Could you check a few things on this model? Use its own coordinates, in mm. Face numbers are marked on the shaded views. A direction names the side the tool comes from. Give positions to 0.01 mm unless a question says otherwise; leave off trailing zeros. Loops run counter-clockwise (first coordinate to the right, second up) from the corner with the lowest first, then second, coordinate; pieces in that order, holes last. Notation, with made-up numbers: M 81.5,12.25 L 113.5,12.25 A32 ccw 113.5,43.25 Z; hole C 80.5,62.25 d4. An arc over 180 degrees is marked long. Use CSV: the item, a comma, the result in double quotes.
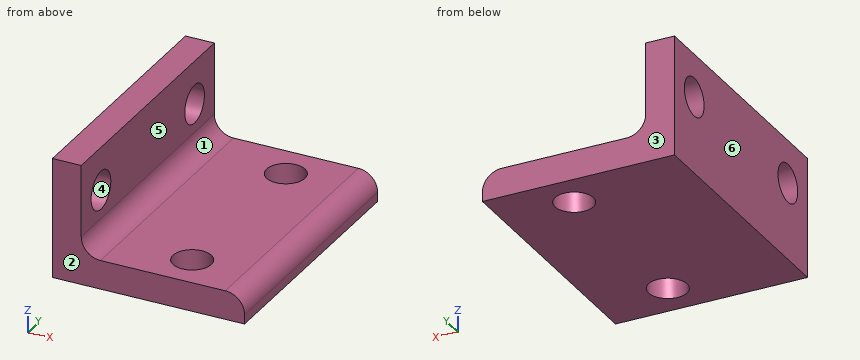
```python
from build123d import *

# Parameters (mm, degrees)
F1_DEPTH = 54
F2_R     = 4
F4_D     = 8
F4_DEPTH = 25
F6_D     = 8
F6_DEPTH = 25


with BuildPart() as f1:
    # F0 (on Front) → F1 (new body)
    with BuildSketch(Plane.XZ):
        Polygon((0, 25), (0, 0), (40, 0), (40, 6), (6, 6), (6, 25), align=None)
    extrude(amount=F1_DEPTH)

    # F2
    f2_edges = [f1.edges().sort_by_distance(p)[0] for p in [
        (40, -27, 6),
        (6, -27, 6),
    ]]
    fillet(f2_edges, radius=F2_R)

    # F4
    with Locations(Plane(origin=(0, 0, 0), x_dir=(0, -1, 0), z_dir=(-1, 0, 0))):
        with Locations((8, 16), (46, 16)):
            Hole(F4_D / 2, depth=F4_DEPTH)

    # F6
    with Locations(Plane(origin=(0, 0, 0), x_dir=(1, 0, 0), z_dir=(0, 0, -1))):
        with Locations((25, 8), (25, 46), (25, 46)):
            Hole(F6_D / 2, depth=F6_DEPTH)


solid = f1.part
```
1. I want a section at C-C, the plane z = 16. List the corners of the cut face in (x, y) for me, then the cut area to 3 significant figures.
Outcome:
outline,"M 0,-54 L 6,-54 L 6,-50 L 0,-50 Z; M 0,-42 L 6,-42 L 6,-12 L 0,-12 Z; M 0,-4 L 6,-4 L 6,0 L 0,0 Z"
area,"228 mm2"
2. Which directions (+Z, -Z, +X, -X, +Y, -Y) give clear straight access to the entire face, cutting with the end or side of a thin tool? Please do the marked faces 5 and 6.
Outcome:
face 5,"+Z, +X, +Y, -Y"
face 6,"+Z, -Z, -X, +Y, -Y"
3. I'm going to push flat-ended pins straight in: pin 1 Ø5 at (y, z) = (-33, 15.5) entering from +X; pin 2 Ø10.5 at (x, y) = (25, -8) entering from +Z; pin 3 Ø6.5 at (x, y) = (25, -46) entering from -Z. Where does each tip first touch, or does it pass through?
Outcome:
pin 1,"x = 6"
pin 2,"z = 6"
pin 3,"through"
4. I want a section at D-D, the plane x = 3. List the corners of the cut face in (y, z) for me, then the cut area to 3 significant figures.
Outcome:
outline,"M -54,0 L 0,0 L 0,25 L -54,25 Z; hole C -46,16 d8; hole C -8,16 d8"
area,"1,250 mm2"
5. I want a section at A-A, the plane x = 25. List the corners of the cut face in (y, z) for me.
Outcome:
outline,"M -54,0 L -50,0 L -50,6 L -54,6 Z; M -42,0 L -12,0 L -12,6 L -42,6 Z; M -4,0 L 0,0 L 0,6 L -4,6 Z"
6. Please list where these lines run through material, in increasing order: line 1 (Y direction, x = 25, z = 2.05); line 2 (Z direction, x = 3.6, y = -8); line 3 (Z direction, x = 25, y = -50.5).
Outcome:
line 1,"-54 to -50, -42 to -12, -4 to 0"
line 2,"0 to 12, 20 to 25"
line 3,"0 to 6"
7. If we mould it in two halves opening along Y, with no side actions, what happens to the marked faces 1, 2, 3 and 4? For each: +Y half, -Y half, draft (parallel to the pull), parting line (faces both ways), or undercut.
Outcome:
face 1,"draft"
face 2,"-Y half"
face 3,"+Y half"
face 4,"undercut"
8. I want a section at B-B, the plane y = -46. List the corners of the cut face in (x, z) for me.
Outcome:
outline,"M 0,0 L 21,0 L 21,6 L 10,6 A4 cw 6,10 L 6,12 L 0,12 Z; M 0,20 L 6,20 L 6,25 L 0,25 Z; M 29,0 L 40,0 L 40,2 A4 ccw 36,6 L 29,6 Z"
